Read the model definition and answer for the solid it produces. Units are mm, in the model's axes. Face numbers are marked on the shaded views. A direction names the side the tool comes from. Coordinates: 2 decimals unless noted, no trailing zeros. Order: outer loops, then holes, each group sorted by start corner. A loop starts at its lowest first (then second) coordinate and runs counter-clockwise, first axis right, second up. Notation, with made-up numbers: (39.5, 17) - (50.5, 17) arc R25 ccw to (50.5, 51) - close; hole circle Ø1 at (26, 41). An arc over 180 degrees is marked (long way). Use one line per item in the form item = value. Start each with the question number.
from build123d import *

# Parameters (mm, degrees)
SKETCH_1_R          = 2.25
EXTRUDE_2_DEPTH     = 20
SKETCH_7_W          = 2.4
SKETCH_7_H          = 2.4
CUT_EXTRUDE_3_DEPTH = 2.5
SKETCH_9_R          = 3
EXTRUDE_4_DEPTH     = 1
SKETCH_10_W         = 4
SKETCH_10_H         = 4
EXTRUDE_5_DEPTH     = 2
CUT_EXTRUDE_START   = -20
SKETCH_12_OUTSIDE_W = 12.904
SKETCH_12_OUTSIDE_H = 12.904
SKETCH_12_OUTSIDE_R = 1
CUT_EXTRUDE_4_DEPTH = 16.5


with BuildPart() as part:
    # 草图1 → 凸台-拉伸2 (new body)
    with BuildSketch(Plane.XY):
        Circle(SKETCH_1_R)
    extrude(amount=EXTRUDE_2_DEPTH)

    # 草图7 → 切除-拉伸3 (cut)
    with BuildSketch(Plane.XY):
        Rectangle(SKETCH_7_W, SKETCH_7_H)
    extrude(amount=CUT_EXTRUDE_3_DEPTH, mode=Mode.SUBTRACT)

    # 草图9 → 凸台-拉伸4 (add)
    with BuildSketch(Plane.XY.offset(20)):
        Circle(SKETCH_9_R)
    extrude(amount=EXTRUDE_4_DEPTH)

    # 草图10 → 凸台-拉伸5 (add)
    with BuildSketch(Plane.XY.offset(21)):
        Rectangle(SKETCH_10_W, SKETCH_10_H)
    extrude(amount=EXTRUDE_5_DEPTH)

    # 草图12 outside → 切除-拉伸4 (cut)
    with BuildSketch(Plane(origin=(0, 0, 0), x_dir=(-1, 0, 0), z_dir=(0, 0, -1)).offset(CUT_EXTRUDE_START)):
        Rectangle(SKETCH_12_OUTSIDE_W, SKETCH_12_OUTSIDE_H)
        Circle(SKETCH_12_OUTSIDE_R, mode=Mode.SUBTRACT)
    extrude(amount=CUT_EXTRUDE_4_DEPTH, mode=Mode.SUBTRACT)


solid = part.part
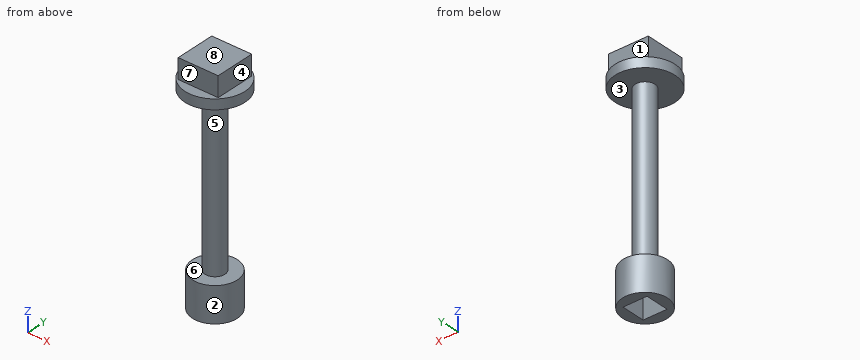
Q1. For a pull along Z with two mould halves and no side action, classify the marked faces 5, 6, 7 and 8 as +Z half, -Z half, draft (parallel to the pull), parting line (faces both ways), or undercut.
Q2. Given P1, Ø0.7, axis at x = -0.5, y = 0.5, coming from the -Z side; P2, Ø2, axis at x = 1, y = 2.5, coming from the +Z side; P3, Ø1, axis at x = 1, z = 22.5, coming from the -Y side; P4, Ø1.9, axis at y = -0.5, z = 2, coming from the +X side, each flat-ended and moving along its own axis, determine where each tip first touches the part or whether it passes through.
Q3. A cutting plane is placed at B-B (y = 0). Give the vertices of the cut face in (x, z).
Q4. A cutting plane is placed at A-A (x = 1.5). Give the vertices of the cut face in (y, z), then the cut area to 3 significant figures.
Q5. Which of the six approach directions +Z, -Z, +X, -X, +Y, -Y give full straight-line access (tool end or side, diameter ignored) to the marked faces 1, 2, 3 and 4?
Q6. A cutting plane is placed at D-D (z = 20.5). Give the vertices of the cut face in (x, y), then the cut area to 3 significant figures.
Q7. Consider probe 1 along Z at (x, y) = (-0.25, 1.45); probe 2 along X at (y, z) = (-0.1, 17.25); probe 3 along Y at (x, z) = (0.45, 19.75). Determine where each line is inside the solid, lowest interval first.
Result sheet:
q1.face_5 = undercut
q1.face_6 = undercut
q1.face_7 = draft
q1.face_8 = +Z half
q2.P1 = 2.5
q2.P2 = 23
q2.P3 = -2
q2.P4 = 2.25
q3.outline = (-3, 20) - (-1, 20) - (-1, 3.5) - (-2.25, 3.5) - (-2.25, 0) - (-1.2, 0) - (-1.2, 2.5) - (1.2, 2.5) - (1.2, 0) - (2.25, 0) - (2.25, 3.5) - (1, 3.5) - (1, 20) - (3, 20) - (3, 21) - (2, 21) - (2, 23) - (-2, 23) - (-2, 21) - (-3, 21) - close
q4.outline = (-2.6, 20) - (2.6, 20) - (2.6, 21) - (2, 21) - (2, 23) - (-2, 23) - (-2, 21) - (-2.6, 21) - close; (-1.68, 0) - (1.68, 0) - (1.68, 3.5) - (-1.68, 3.5) - close
q4.area = 24.9 mm^2
q5.face_1 = +Z, +X, -X, +Y
q5.face_2 = -Z
q5.face_3 = none
q5.face_4 = +Z, +X, +Y, -Y
q6.outline = circle Ø6 at (0, 0)
q6.area = 28.3 mm^2
q7.probe_1 = 0 to 3.5, 20 to 23
q7.probe_2 = -0.99 to 0.99
q7.probe_3 = -0.89 to 0.89
